The listing builds one solid part. Answer for the finished solid, in the listing's coordinates (mm). Face numbers are marked on the shaded views. A direction names the side the tool comes from. Round coordinates to 2 decimals unless told otherwise and drop trailing zeros. Loops run counter-clockwise (first coordinate to the right, second up) from the corner with the lowest first, then second, coordinate; pieces in that order, holes last. Notation, with made-up numbers: (54.25, 6) - (77.25, 6) arc R18 cw to (77.25, 21) - close; hole circle Ø2 at (7, -11). An arc over 180 degrees is marked (long way). Write item = value, one per line. Start each with the question number.
1) Section D-D, the plane y = -3.25 is taken. Determine the outline of the cut face in (x, z).
2) A tool of negligible diameter and unlimited length cuts with its end or side. For the marked faces 4 and 5, from which of +Z, -Z, +X, -X, +Y, -Y can it reach the whole face along a straight path? Write none if from no direction.
3) Section C-C, the plane x = 6.75 is taken. Determine the outline of the cut face in (y, z) (3 decimals), and give its area (3 significant figures).
4) Section B-B, the plane z = 0 is taken. Determine the outline of the cut face in (x, y) (3 decimals).
5) Straight lines are drawn through the part: line 1 along X through (y, z) = (1.25, 1.75); line 2 along Z through (x, y) = (3, -10.9) (3 decimals); line 3 along Z through (x, y) = (7.75, -10.9) (3 decimals). For each, find the intervals that lie inside material, in ascending order.
6) For a pull along X with two mould halves and no side action, classify the marked faces 1, 2 and 3 as released by +X, released by -X, zero draft, split by the parting line, or undercut.
7) Section A-A, the plane y = -10.9 is taken. Determine the outline of the cut face in (x, z) (3 decimals), and give its area (3 significant figures).
8) Given pin 1 Ø1.5 at (y, z) = (-9.5, -11) entering from +X; pin 2 Ø3 at (x, z) = (-2, -8) entering from -Y; pin 3 Ø2 at (x, z) = (4, 9) entering from -Y, each flat-ended and moving along its own axis, determine where each tip first touches the part or whether it passes through.
from build123d import *

# Parameters (mm, degrees)
CUT_EXTRUDE1_DEPTH      = 36.02253703
CUT_EXTRUDE1_DEPTH_BACK = 36.02253703
SKETCH4_R               = 3.175


with BuildPart() as part:
    # Sketch1 → Revolve1 (revolve)
    with BuildSketch(Plane.XY, mode=Mode.PRIVATE) as revolve1_sk:
        Polygon((-3.33, 0), (3.33, 0), (3.33, 4), (4.83, 4), (4.83, -0.900000061), (13.58, -0.900000061), (13.58, -10.9), (-4.83, -10.9), (-4.83, 4), (-3.33, 4), align=None)
    revolve(revolve1_sk.sketch.rotate(Axis((-4.83, -10.9, 0), (1, 0, 0)), 180), axis=Axis((-4.83, -10.9, 0), (1, 0, 0)))

    # Sketch4 → Cut-Extrude1 (cut, two sides: drawn at the far end of the back side and taken through both)
    with BuildSketch(Plane(origin=(13.58, 0, 0), x_dir=(0, 0, -1), z_dir=(1, 0, 0)).offset(-CUT_EXTRUDE1_DEPTH_BACK)):
        with Locations(Location((0, -10.9, 0), (0, 0, 90))):
            Circle(SKETCH4_R)
    extrude(amount=CUT_EXTRUDE1_DEPTH + CUT_EXTRUDE1_DEPTH_BACK, mode=Mode.SUBTRACT)


solid = part.part
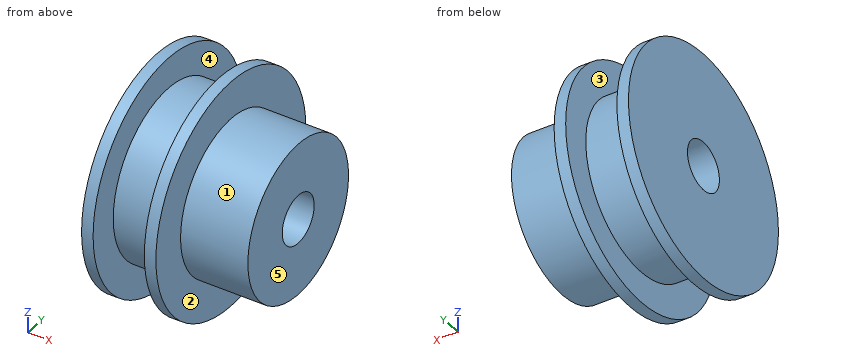
Geometry check:
q1.outline = (-4.83, -12.79) - (-3.33, -12.79) - (-3.33, -7.76) - (3.33, -7.76) - (3.33, -12.79) - (4.83, -12.79) - (4.83, -6.44) - (13.58, -6.44) - (13.58, 6.44) - (4.83, 6.44) - (4.83, 12.79) - (3.33, 12.79) - (3.33, 7.76) - (-3.33, 7.76) - (-3.33, 12.79) - (-4.83, 12.79) - close
q2.face_4 = none
q2.face_5 = +Z, -Z, +X, +Y, -Y
q3.outline = circle Ø20 at (-10.9, 0); hole circle Ø6.35 at (-10.9, 0)
q3.area = 282 mm2
q4.outline = (-4.83, -25.8) - (-3.33, -25.8) - (-3.33, -21.8) - (3.33, -21.8) - (3.33, -25.8) - (4.83, -25.8) - (4.83, -20.9) - (13.58, -20.9) - (13.58, -14.075) - (-4.83, -14.075) - close; (-4.83, -7.725) - (13.58, -7.725) - (13.58, -0.9) - (4.83, -0.9) - (4.83, 4) - (3.33, 4) - (3.33, 0) - (-3.33, 0) - (-3.33, 4) - (-4.83, 4) - close
q5.line_1 = -4.83 to -3.33, 3.33 to 4.83
q5.line_2 = -10.9 to -3.175, 3.175 to 10.9
q5.line_3 = -10 to -3.175, 3.175 to 10
q6.face_1 = zero draft
q6.face_2 = released by +X
q6.face_3 = undercut
q7.outline = (-4.83, -14.9) - (-3.33, -14.9) - (-3.33, -10.9) - (3.33, -10.9) - (3.33, -14.9) - (4.83, -14.9) - (4.83, -10) - (13.58, -10) - (13.58, -3.175) - (-4.83, -3.175) - close; (-4.83, 3.175) - (13.58, 3.175) - (13.58, 10) - (4.83, 10) - (4.83, 14.9) - (3.33, 14.9) - (3.33, 10.9) - (-3.33, 10.9) - (-3.33, 14.9) - (-4.83, 14.9) - close
q7.area = 293 mm2
q8.pin_1 = 4.83
q8.pin_2 = -23.89
q8.pin_3 = -23.47
